Source: CAD feature listing. Evaluate the final solid. Frame: model axes, mm. A direction names the side the tool comes from. Round coordinates to 2 decimals unless told otherwise and drop trailing zeros. Order: outer loops, then holes, each group sorted by start corner. A loop starts at its lowest first (then second) coordinate and runs counter-clockwise, first axis right, second up. Notation, with made-up numbers: (-20.75, 10.25) - (5.25, 10.25) arc R14 cw to (5.25, 29.25) - close; hole circle Ø4 at (79.5, -38). An arc over 180 degrees is marked (long way). Return JSON: item names as keys, results as strings. Group by question number.
1) Contact query for a flat-ended pin moving along its axis: P1, Ø2.5, axis at y = -13, z = 2.5, coming from the +X side (3 decimals). Output: stop coordinate, or through.
2) Section B-B, the plane x = 0. Return loops of the section in (y, z) (3 decimals).
3) Access query for faces 1 (the flat face through (0, -20.405, 3)), 2 (the flat face through (1.905, -14, 3)). Directions: +Z, -Z, +X, -X, +Y, -Y. A direction counts if a zero-diameter tool reaches every point of the face in a straight line with its end or side. Return the directions, or none.
4) Ray query, line 1 (Y direction, x = 0, z = 2.5) (3 decimals); line 2 (Y direction, x = 0.5, z = 2.85) (3 decimals); line 3 (Y direction, x = 9, z = 2.8). Return the intervals inside material, ascending. Write a range as from..to.
5) Mould query, pull axis Y, two halves, no side actions, for faces 3 (the cylindrical face through (-0.14, 17.88, 2.5)), 4 (the flat face through (6, -6.833, 3)), 5 (the flat face through (10.795, 8, 3)). Classes: pulls with the +Y half, pulls with the -Y half, needs draft (parallel to the pull), parting line crosses it, or undercut.
6) Section C-C, the plane z = 1.7. Return loops of the section in (x, y) (3 decimals).
7) Section A-A, the plane y = -18.5. Return loops of the section in (x, z) (3 decimals), plus the area to 3 significant figures.
8) Section D-D, the plane y = -13.5. Return loops of the section in (x, z) (3 decimals), plus the area to 3 significant figures.
```python
from build123d import *

# Parameters (mm, degrees)
SKETCH_R        = 0.635
PAD_DEPTH       = 5.08
CHAMFER_SIZE    = 1
CHAMFER001_SIZE = 1


with BuildPart() as part:
    # Sketch → Pad (new body)
    with BuildSketch(Plane.XY):
        Polygon((-1.905, 23.0759), (-1.905, -20.405), (1.905, -20.405), (1.905, -6.833036), (10.795, -6.833036), (10.795, 23.0759), align=None)
        with Locations((0, 18.5)):
            Circle(SKETCH_R, mode=Mode.SUBTRACT)
        with Locations((0, -18.5)):
            Circle(SKETCH_R, mode=Mode.SUBTRACT)
    extrude(amount=PAD_DEPTH)

    # Chamfer
    chamfer_edges = [part.edges().sort_by_distance(p)[0] for p in [
        (-1.905, 1.33545, 0),
    ]]
    chamfer(chamfer_edges, length=CHAMFER_SIZE)

    # Chamfer001
    chamfer001_edges = [part.edges().sort_by_distance(p)[0] for p in [
        (1.905, -6.833036, 2.54),
        (10.795, -6.833036, 2.54),
        (10.795, 23.0759, 2.54),
    ]]
    chamfer(chamfer001_edges, length=CHAMFER001_SIZE)


solid = part.part
```
Geometry check:
{
 "1": {"P1": "x = 1.905"},
 "2": {"outline": "(-20.405, 0) - (-19.135, 0) - (-19.135, 5.08) - (-20.405, 5.08) - close; (-17.865, 0) - (17.865, 0) - (17.865, 5.08) - (-17.865, 5.08) - close; (19.135, 0) - (23.076, 0) - (23.076, 5.08) - (19.135, 5.08) - close"},
 "3": {"face 1": "+Z, -Z, +X, -X, -Y", "face 2": "+Z, -Z, +X, -Y"},
 "4": {"line 1": "-20.405..-19.135, -17.865..17.865, 19.135..23.076", "line 2": "-20.405..-18.891, -18.109..18.109, 18.891..23.076", "line 3": "-6.83..23.08"},
 "5": {"face 3": "undercut", "face 4": "pulls with the -Y half", "face 5": "needs draft"},
 "6": {"outline": "(-1.905, -20.405) - (1.905, -20.405) - (1.905, -7.833) - (2.905, -6.833) - (9.795, -6.833) - (10.795, -5.833) - (10.795, 22.076) - (9.795, 23.076) - (-1.905, 23.076) - close; hole circle Ø1.27 at (0, -18.5); hole circle Ø1.27 at (0, 18.5)"},
 "7": {"outline": "(-1.905, 1) - (-0.905, 0) - (-0.635, 0) - (-0.635, 5.08) - (-1.905, 5.08) - close; (0.635, 0) - (1.905, 0) - (1.905, 5.08) - (0.635, 5.08) - close", "area": "12.4 mm2"},
 "8": {"outline": "(-1.905, 1) - (-0.905, 0) - (1.905, 0) - (1.905, 5.08) - (-1.905, 5.08) - close", "area": "18.9 mm2"}
}
